Work out the finished part from the listing and answer in its coordinate system (mm). Coordinates: 2 decimals unless noted, no trailing zeros. Order: outer loops, then holes, each group sorted by start corner. A loop starts at its lowest first (then second) coordinate and runs counter-clockwise, first axis right, second up. Notation, with made-up numbers: (23.25, -31.5) -> (43.25, -31.5) arc R5 ccw to (43.25, -24.5) -> close; hole circle Ø1 at (62, -30). An arc over 180 degrees is marked (long way). Use one line per item in the form item = value.
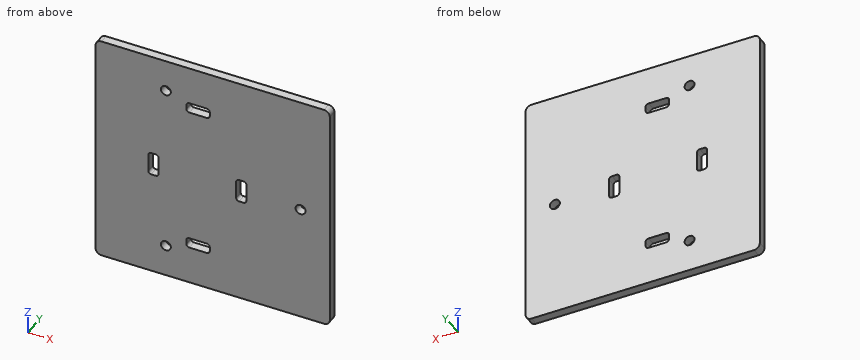
from build123d import *

# Parameters (mm, degrees)
SKETCH1_W           = 80
SKETCH1_H           = 80
BOSS_EXTRUDE1_DEPTH = 3
SKETCH5_R           = 1.7
SKETCH5_W           = 3.5
SKETCH5_H           = 8
SKETCH5_W_2         = 8
SKETCH5_H_2         = 3.5
CUT_EXTRUDE5_DEPTH  = 3
FILLET1_R           = 1
FILLET2_R           = 1
FILLET3_R           = 2


with BuildPart() as part:
    # Sketch1 → Boss-Extrude1 (new body)
    with BuildSketch(Plane(origin=(0, 0, 0), x_dir=(1, 0, 0), z_dir=(0, 1, 0))):
        Rectangle(SKETCH1_W, SKETCH1_H)
    extrude(amount=BOSS_EXTRUDE1_DEPTH)

    # Sketch5 → Cut-Extrude5 (cut)
    with BuildSketch(Plane(origin=(0, 0, 0), x_dir=(1, 0, 0), z_dir=(0, 1, 0))):
        with Locations(Location((30, 0, 0), (0, 0, 270))):
            Circle(SKETCH5_R)
        with Locations(Location((-16, 29, 0), (0, 0, 270))):
            Circle(SKETCH5_R)
        with Locations(Location((-16, -29, 0), (0, 0, 270))):
            Circle(SKETCH5_R)
        with Locations((9.75, 0)):
            Rectangle(SKETCH5_W, SKETCH5_H)
        with Locations((-20.25, 0)):
            Rectangle(SKETCH5_W, SKETCH5_H)
        with Locations((-5, 25.25)):
            Rectangle(SKETCH5_W_2, SKETCH5_H_2)
        with Locations((-5, -25.25)):
            Rectangle(SKETCH5_W_2, SKETCH5_H_2)
    extrude(amount=CUT_EXTRUDE5_DEPTH, mode=Mode.SUBTRACT)

    # Fillet1
    fillet1_edges = [part.edges().sort_by_distance(p)[0] for p in [
        (11.5, 1.5, 4),
        (11.5, 1.5, -4),
        (8, 1.5, -4),
        (8, 1.5, 4),
    ]]
    fillet(fillet1_edges, radius=FILLET1_R)

    # Fillet2
    fillet2_edges = [part.edges().sort_by_distance(p)[0] for p in [
        (-1, 1.5, 27),
        (-1, 1.5, 23.5),
        (-9, 1.5, 23.5),
        (-9, 1.5, 27),
        (-1, 1.5, -23.5),
        (-1, 1.5, -27),
        (-9, 1.5, -27),
        (-9, 1.5, -23.5),
        (-18.5, 1.5, 4),
        (-18.5, 1.5, -4),
        (-22, 1.5, -4),
        (-22, 1.5, 4),
    ]]
    fillet(fillet2_edges, radius=FILLET2_R)

    # Fillet3
    fillet3_edges = [part.edges().sort_by_distance(p)[0] for p in [
        (40, 1.5, 40),
        (-40, 1.5, 40),
        (-40, 1.5, -40),
        (40, 1.5, -40),
    ]]
    fillet(fillet3_edges, radius=FILLET3_R)


solid = part.part
(1) Section C-C on z = 29 is taken. Write down the section's boundary in (x, y).
Data:
outline = (-40, 0) -> (-17.7, 0) -> (-17.7, 3) -> (-40, 3) -> close; (-14.3, 0) -> (40, 0) -> (40, 3) -> (-14.3, 3) -> close
(2) Section D-D on x = 30 is taken. Write down the section's boundary in (y, z).
Data:
outline = (0, -40) -> (3, -40) -> (3, -1.7) -> (0, -1.7) -> close; (0, 1.7) -> (3, 1.7) -> (3, 40) -> (0, 40) -> close
(3) Straight lines are drawn through the part: line 1 along Z through (x, y) = (-14.5, 1.7); line 2 along X through (y, z) = (1.4, -29); line 3 along Z through (x, y) = (10, 2.3). For each, find the intervals that lie inside material, in ascending order.
Data:
line_1 = -40 to -29.8, -28.2 to 28.2, 29.8 to 40
line_2 = -40 to -17.7, -14.3 to 40
line_3 = -40 to -4, 4 to 40
(4) This flat-tipped pin is pushed along its axis until it touches: P1, Ø2.5, axis at x = -16, z = 29, coming from the +Y side. Where does it stop, or does it pass through?
Data:
P1 = through
(5) Section B-B on x = -7 is taken. Write down the section's boundary in (y, z).
Data:
outline = (0, -40) -> (3, -40) -> (3, -27) -> (0, -27) -> close; (0, -23.5) -> (3, -23.5) -> (3, 23.5) -> (0, 23.5) -> close; (0, 27) -> (3, 27) -> (3, 40) -> (0, 40) -> close
(6) Section A-A on z = 0 is taken. Write down the section's boundary in (x, y).
Data:
outline = (-40, 0) -> (-22, 0) -> (-22, 3) -> (-40, 3) -> close; (-18.5, 0) -> (8, 0) -> (8, 3) -> (-18.5, 3) -> close; (11.5, 0) -> (28.3, 0) -> (28.3, 3) -> (11.5, 3) -> close; (31.7, 0) -> (40, 0) -> (40, 3) -> (31.7, 3) -> close
